from build123d import *

# Parameters (mm, degrees)
SKETCH2_R           = 50
SKETCH2_R_2         = 39
BOSS_EXTRUDE1_DEPTH = 5
SKETCH3_R           = 47
SKETCH3_R_2         = 3
SKETCH3_R_3         = 39
BOSS_EXTRUDE2_DEPTH = 4
SKETCH4_R           = 39
SKETCH4_R_2         = 37
BOSS_EXTRUDE3_DEPTH = 1
SKETCH6_R           = 5
SKETCH6_R_2         = 2
BOSS_EXTRUDE4_DEPTH = 5
FILLET1_R           = 5
SKETCH7_R           = 3.6
CUT_EXTRUDE1_DEPTH  = 3
SKETCH8_R           = 3.15
CUT_EXTRUDE2_DEPTH  = 4
SKETCH9_R           = 3.15
CUT_EXTRUDE3_DEPTH  = 6.6
SKETCH10_R          = 57.5
SKETCH10_R_2        = 47.5
CUT_EXTRUDE4_DEPTH  = 5
SKETCH11_R          = 47.5
SKETCH11_R_2        = 46.4
CUT_EXTRUDE5_DEPTH  = 4
SKETCH12_R          = 2
BOSS_EXTRUDE7_DEPTH = 5
FILLET3_R           = 10
SKETCH14_R          = 3.6
CUT_EXTRUDE8_DEPTH  = 2


with BuildPart() as part:
    # Sketch2 → Boss-Extrude1 (new body)
    with BuildSketch(Plane.XY):
        Circle(SKETCH2_R)
        Circle(SKETCH2_R_2, mode=Mode.SUBTRACT)
    extrude(amount=BOSS_EXTRUDE1_DEPTH)

    # Sketch3 → Boss-Extrude2 (add)
    with BuildSketch(Plane(origin=(0, 0, 0), x_dir=(-1, 0, 0), z_dir=(0, 0, -1))):
        Circle(SKETCH3_R)
        with Locations((-43, 0)):
            Circle(SKETCH3_R_2, mode=Mode.SUBTRACT)
        Circle(SKETCH3_R_3, mode=Mode.SUBTRACT)
        with Locations((-32.939911054, 27.639867217)):
            Circle(SKETCH3_R_2, mode=Mode.SUBTRACT)
        with Locations((-7.46687164, 42.34673338)):
            Circle(SKETCH3_R_2, mode=Mode.SUBTRACT)
        with Locations((21.5, 37.239092363)):
            Circle(SKETCH3_R_2, mode=Mode.SUBTRACT)
        with Locations((40.406782694, 14.706866163)):
            Circle(SKETCH3_R_2, mode=Mode.SUBTRACT)
        with Locations((40.406782694, -14.706866163)):
            Circle(SKETCH3_R_2, mode=Mode.SUBTRACT)
        with Locations((21.5, -37.239092363)):
            Circle(SKETCH3_R_2, mode=Mode.SUBTRACT)
        with Locations((-7.46687164, -42.34673338)):
            Circle(SKETCH3_R_2, mode=Mode.SUBTRACT)
        with Locations((-32.939911054, -27.639867217)):
            Circle(SKETCH3_R_2, mode=Mode.SUBTRACT)
    extrude(amount=BOSS_EXTRUDE2_DEPTH)

    # Sketch4 → Boss-Extrude3 (add)
    with BuildSketch(Plane(origin=(0, 0, -4), x_dir=(-1, 0, 0), z_dir=(0, 0, -1))):
        Circle(SKETCH4_R)
        Circle(SKETCH4_R_2, mode=Mode.SUBTRACT)
    extrude(amount=-BOSS_EXTRUDE3_DEPTH)

    # Sketch6 → Boss-Extrude4 (add)
    with BuildSketch(Plane.XY.offset(5)):
        with Locations((52, 0)):
            Circle(SKETCH6_R)
        with Locations((52, 0)):
            Circle(SKETCH6_R_2, mode=Mode.SUBTRACT)
        with Locations((-52, 0)):
            Circle(SKETCH6_R)
        with Locations((-52, 0)):
            Circle(SKETCH6_R_2, mode=Mode.SUBTRACT)
        with Locations((0, 52)):
            Circle(SKETCH6_R)
        with Locations((0, 52)):
            Circle(SKETCH6_R_2, mode=Mode.SUBTRACT)
        with Locations((0, -52)):
            Circle(SKETCH6_R)
        with Locations((0, -52)):
            Circle(SKETCH6_R_2, mode=Mode.SUBTRACT)
    extrude(amount=-BOSS_EXTRUDE4_DEPTH)

    # Fillet1
    fillet1_edges = [part.edges().sort_by_distance(p)[0] for p in [
        (49.798076923, -4.489046086, 2.5),
        (49.798076923, 4.489046086, 2.5),
        (-49.798076923, 4.489046086, 2.5),
        (-49.798076923, -4.489046086, 2.5),
        (4.489046086, 49.798076923, 2.5),
        (-4.489046086, 49.798076923, 2.5),
        (-4.489046086, -49.798076923, 2.5),
        (4.489046086, -49.798076923, 2.5),
    ]]
    fillet(fillet1_edges, radius=FILLET1_R)

    # Sketch7 → Cut-Extrude1 (cut)
    with BuildSketch(Plane.XY.offset(5)):
        with Locations((52, 0)):
            Circle(SKETCH7_R)
        with Locations((0, 52)):
            Circle(SKETCH7_R)
        with Locations((-52, 0)):
            Circle(SKETCH7_R)
        with Locations((0, -52)):
            Circle(SKETCH7_R)
    extrude(amount=-CUT_EXTRUDE1_DEPTH, mode=Mode.SUBTRACT)

    # Sketch8 → Cut-Extrude2 (cut)
    with BuildSketch(Plane(origin=(0, 0, -4), x_dir=(-1, 0, 0), z_dir=(0, 0, -1))):
        with Locations((-32.939911054, 27.639867217)):
            Circle(SKETCH8_R)
        with Locations((-43, 0)):
            Circle(SKETCH8_R)
        with Locations((-7.46687164, 42.34673338)):
            Circle(SKETCH8_R)
        with Locations((21.5, 37.239092363)):
            Circle(SKETCH8_R)
        with Locations((40.406782694, 14.706866163)):
            Circle(SKETCH8_R)
        with Locations((40.406782694, -14.706866163)):
            Circle(SKETCH8_R)
        with Locations((21.5, -37.239092363)):
            Circle(SKETCH8_R)
        with Locations((-7.46687164, -42.34673338)):
            Circle(SKETCH8_R)
        with Locations((-32.939911054, -27.639867217)):
            Circle(SKETCH8_R)
    extrude(amount=-CUT_EXTRUDE2_DEPTH, mode=Mode.SUBTRACT)

    # Sketch9 → Cut-Extrude3 (cut)
    with BuildSketch(Plane(origin=(0, 0, -4), x_dir=(-1, 0, 0), z_dir=(0, 0, -1))):
        with Locations((-43, 0)):
            Circle(SKETCH9_R)
        with Locations((-32.939911054, 27.639867217)):
            Circle(SKETCH9_R)
        with Locations((-7.46687164, 42.34673338)):
            Circle(SKETCH9_R)
        with Locations((21.5, 37.239092363)):
            Circle(SKETCH9_R)
        with Locations((40.406782694, 14.706866163)):
            Circle(SKETCH9_R)
        with Locations((40.406782694, -14.706866163)):
            Circle(SKETCH9_R)
        with Locations((21.5, -37.239092363)):
            Circle(SKETCH9_R)
        with Locations((-7.46687164, -42.34673338)):
            Circle(SKETCH9_R)
        with Locations((-32.939911054, -27.639867217)):
            Circle(SKETCH9_R)
    extrude(amount=-CUT_EXTRUDE3_DEPTH, mode=Mode.SUBTRACT)

    # Sketch10 → Cut-Extrude4 (cut)
    with BuildSketch(Plane(origin=(0, 0, 0), x_dir=(-1, 0, 0), z_dir=(0, 0, -1))):
        Circle(SKETCH10_R)
        Circle(SKETCH10_R_2, mode=Mode.SUBTRACT)
    extrude(amount=-CUT_EXTRUDE4_DEPTH, mode=Mode.SUBTRACT)

    # Sketch11 → Cut-Extrude5 (cut)
    with BuildSketch(Plane(origin=(0, 0, -4), x_dir=(-1, 0, 0), z_dir=(0, 0, -1))):
        Circle(SKETCH11_R)
        Circle(SKETCH11_R_2, mode=Mode.SUBTRACT)
    extrude(amount=-CUT_EXTRUDE5_DEPTH, mode=Mode.SUBTRACT)

    # Sketch12 → Boss-Extrude7 (add)
    with BuildSketch(Plane.XY.offset(5)):
        with BuildLine():
            ThreePointArc((47.3125, -4.216318744), (55, 0), (47.3125, 4.216318744))
            ThreePointArc((47.3125, 4.216318744), (47.5, 0), (47.3125, -4.216318744))
        make_face()
        with Locations((50, 0)):
            Circle(SKETCH12_R, mode=Mode.SUBTRACT)
        with BuildLine():
            ThreePointArc((-4.216318744, 47.3125), (0, 47.5), (4.216318744, 47.3125))
            ThreePointArc((4.216318744, 47.3125), (0, 55), (-4.216318744, 47.3125))
        make_face()
        with Locations((0, 50)):
            Circle(SKETCH12_R, mode=Mode.SUBTRACT)
        with BuildLine():
            ThreePointArc((-4.216318744, -47.3125), (0, -55), (4.216318744, -47.3125))
            ThreePointArc((4.216318744, -47.3125), (0, -47.5), (-4.216318744, -47.3125))
        make_face()
        with Locations((0, -50)):
            Circle(SKETCH12_R, mode=Mode.SUBTRACT)
        with BuildLine():
            ThreePointArc((-47.3125, -4.216318744), (-47.5, 0), (-47.3125, 4.216318744))
            ThreePointArc((-47.3125, 4.216318744), (-55, 0), (-47.3125, -4.216318744))
        make_face()
        with Locations((-50, 0)):
            Circle(SKETCH12_R, mode=Mode.SUBTRACT)
    extrude(amount=-BOSS_EXTRUDE7_DEPTH)

    # Fillet3
    fillet3_edges = [part.edges().sort_by_distance(p)[0] for p in [
        (47.3125, -4.216318744, 2.5),
        (47.3125, 4.216318744, 2.5),
        (4.216318744, 47.3125, 2.5),
        (-4.216318744, 47.3125, 2.5),
        (-47.3125, 4.216318744, 2.5),
        (-47.3125, -4.216318744, 2.5),
        (-4.216318744, -47.3125, 2.5),
        (4.216318744, -47.3125, 2.5),
    ]]
    fillet(fillet3_edges, radius=FILLET3_R)

    # Sketch14 → Cut-Extrude8 (cut)
    with BuildSketch(Plane.XY.offset(5)):
        with Locations((50, 0)):
            Circle(SKETCH14_R)
        with Locations((0, -50)):
            Circle(SKETCH14_R)
        with Locations((-50, 0)):
            Circle(SKETCH14_R)
        with Locations((0, 50)):
            Circle(SKETCH14_R)
    extrude(amount=-CUT_EXTRUDE8_DEPTH, mode=Mode.SUBTRACT)


solid = part.part
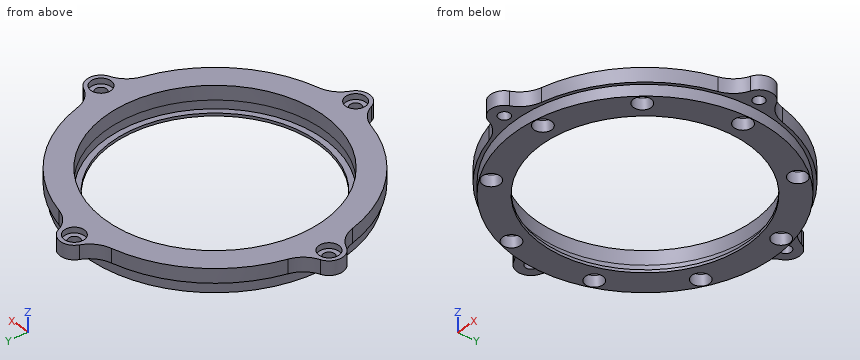
The listing builds one solid part. Answer for the finished solid, in the listing's coordinates (mm). Give positions to 0.01 mm unless a question says otherwise; leave off trailing zeros. Loops run counter-clockwise (first coordinate to the right, second up) from the corner with the lowest first, then second, coordinate; pieces in that order, holes last. Notation, with made-up numbers: (-2.75, 81) - (43.25, 81) arc R22 cw to (43.25, 114) - close; hole circle Ø9 at (8, 75). An arc over 180 degrees is marked (long way). Answer as a JSON object with one key per item and string values.
1. Flat-ended cylindrical pins translate along their axes: pin 1 Ø4.5 at (x, y) = (-50, 0) entering from -Z; pin 2 Ø5 at (x, z) = (-16.5, 1) entering from +Y; pin 3 Ø4 at (x, y) = (32.94, -27.64) entering from -Z; pin 4 Ø10 at (x, y) = (-2.5, 30.5) entering from -Z. Find the tip coordinate at first contact, or state that the pin passes through.
Determined:
{"pin 1": "z = 0", "pin 2": "y = 45.39", "pin 3": "z = 2.6", "pin 4": "through"}
2. A cutting plane is placed at C-C (x = 26.5). Write down the section's boundary in (y, z).
Determined:
{"outline": "(-39.42, 0) - (-38.09, 0) - (-38.09, -4) - (-25.82, -4) - (-25.82, -3) - (-28.61, -3) - (-28.61, 5) - (-39.42, 5) - close; (25.82, -4) - (38.09, -4) - (38.09, 0) - (39.42, 0) - (39.42, 5) - (28.61, 5) - (28.61, -3) - (25.82, -3) - close"}
3. A cutting plane is placed at A-A (x = 0). Give the number of separate pieces and of enclosed holes in the cut face, then the cut area to 3 significant figures.
Determined:
{"separate pieces": "4", "enclosed holes": "0", "area": "170 mm²"}
4. Find the intervals of material crossed by L1, parallel to Y at x = -21, z = -2.5; L2, parallel to Y at x = -19.5, z = 0.75 (3 decimals); L3, parallel to Y at x = 0, z = -3.45, in increasing order. Write a range as [from, to].
Determined:
{"L1": "[-41.38, -40.35], [-34.13, -32.86], [32.86, 34.13], [40.35, 41.38]", "L2": "[-43.313, -39.673], [-34.805, -33.775], [33.775, 34.805], [39.673, 43.313]", "L3": "[-46.4, -37], [37, 46.4]"}
5. A cutting plane is placed at B-B (y = -23). Write down the section's boundary in (x, z).
Determined:
{"outline": "(-41.56, 0) - (-40.3, 0) - (-40.3, -4) - (-28.98, -4) - (-28.98, -3) - (-31.5, -3) - (-31.5, 5) - (-41.56, 5) - close; (28.98, -4) - (40.3, -4) - (40.3, 0) - (41.56, 0) - (41.56, 5) - (31.5, 5) - (31.5, -3) - (28.98, -3) - close"}
